from build123d import *

# Parameters (mm, degrees)
F0_R     = 9.5
F1_DEPTH = 8
F2_R     = 5.2
F4_DEPTH = 7.1
F5_R     = 4.55
F6_DEPTH = 35
F7_R     = 13
F7_R_2   = 4.55
F8_DEPTH = 25


with BuildPart() as f1:
    # F0 (on Top) → F1 (new body)
    with BuildSketch(Plane.XY):
        Circle(F0_R)
    extrude(amount=F1_DEPTH)

    # F2
    f2_edges = [f1.edges().sort_by_distance(p)[0] for p in [
        (-9.5, 0, 8),
    ]]
    fillet(f2_edges, radius=F2_R)

    # F3 (on Top) → F4 (join)
    with BuildSketch(Plane.XY):
        Polygon((4.5, -14.8323969742), (1.3178354695, 15.4438761221), (-1.3178354695, 15.4438761221), (-4.5, -14.8323969742), align=None)
    extrude(amount=F4_DEPTH)

    # F5 (on face) → F6 (join)
    with BuildSketch(Plane(origin=(0, 0, 0), x_dir=(1, 0, 0), z_dir=(0, 0, -1))):
        Circle(F5_R)
    extrude(amount=F6_DEPTH)

    # F7 (on face) → F8 (join)
    with BuildSketch(Plane(origin=(0, 0, -35), x_dir=(1, 0, 0), z_dir=(0, 0, -1))):
        Circle(F7_R)
        Circle(F7_R_2, mode=Mode.SUBTRACT)
    extrude(amount=-F8_DEPTH)


solid = f1.part
Part model, mm, in its own coordinate system. A direction names the side the tool comes from. Give positions to 0.01 mm unless a question says otherwise; leave off trailing zeros. Loops run counter-clockwise (first coordinate to the right, second up) from the corner with the lowest first, then second, coordinate; pieces in that order, holes last.
(1) Pin check, flat tips, straight feed: pin 1 (7 mm diameter, centred on x = -1.5, y = -10.5, fed in from +Z); pin 2 (1.5 mm diameter, centred on y = -7, z = -29.5, fed in from +X); pin 3 (8 mm diameter, centred on x = 1, y = 6, fed in from +Z); pin 4 (1.3 mm diameter, centred on x = 0, y = 13, fed in from +Z). Stop position of each tip, or through.
Return value:
pin 1: stops at z = 7.18
pin 2: stops at x = 11.4
pin 3: stops at z = 8
pin 4: stops at z = 7.1
(2) Pull direction Y, two halves, no side cores. Call faces 4 (the flat face through (4.156, -11.56, 3.5)), 5 (the flat face through (0, -14.832, 4)), 6 (the flat face through (0, 0, -35)): pulls with the +Y half, pulls with the -Y half, needs draft (parallel to the pull), parting line crosses it, or undercut.
Return value:
face 4: undercut
face 5: pulls with the -Y half
face 6: needs draft
(3) Drill centre lines: line 1 along Z through (x, y) = (-0.75, -11); line 2 along Y through (x, z) = (-0.25, -23.5); line 3 along Z through (x, y) = (10, 8). Where is each one in solid material? Low to high.
Return value:
line 1: z = -35 to -10, 0 to 7.1
line 2: y = -13 to 13
line 3: z = -35 to -10
(4) 3-axis set-ups, long thin cutter, end or side, ignore diameter. For faces 1 (the flat face through (-1.66, 12.17, 3.5)), 2 (the cylindrical face through (-9.43, 1.16, 1.38)), 3 (the flat face through (4, -3, 0)): which of +Z, -Z, +X, -X, +Y, -Y reach the whole face in a straight line?
Return value:
face 1: +Z, -X, +Y
face 2: +Z, -X
face 3: none
(5) Band-saw the part on C-C (z = -29.5). Write the cut outline in (x, y).
Return value:
outline: circle Ø26 at (0, 0)
(6) Band-saw the part on B-B (y = -9.5). Write the cut outline in (x, z), and give its area (3 significant figures).
Return value:
outline: (-8.87, -35) - (8.87, -35) - (8.87, -10) - (-8.87, -10) - close; (-3.94, 0) - (3.94, 0) - (3.94, 7.1) - (-3.94, 7.1) - close
area: 500 mm2
(7) Band-saw the part on A-A (y = 10.5). Write the cut outline in (x, z).
Return value:
outline: (-7.66, -35) - (7.66, -35) - (7.66, -10) - (-7.66, -10) - close; (-1.84, 0) - (1.84, 0) - (1.84, 7.1) - (-1.84, 7.1) - close
(8) Band-saw the part on D-D (x = -10). Write the cut outline in (y, z), and give its area (3 significant figures).
Return value:
outline: (-8.31, -35) - (8.31, -35) - (8.31, -10) - (-8.31, -10) - close
area: 415 mm2
